Input: dimensioned drawing with shaded views. Units: mm. Origin: part minimum x, y, z. Coordinates: 2 decimals unless noted, no trailing zeros. Order: outer loops, then holes, each group sorted by start corner. A loop starts at its lowest first (then second) coordinate and runs counter-clockwise, first axis right, second up. Notation, with made-up numbers: (-4, 26) - (30, 26) arc R32 ccw to (30, 58) - close; hole circle Ø11 at (-27.5, -9). An arc over 180 degrees is marked (long way). Answer as CSV lines item,"result". Start each with the question number.
Item 1: Section C-C (x = 167). Output: boundary loops of the cut face in (y, z), and give its area (3 significant figures).
Item 2: Section B-B (z = 4). Output: boundary loops of the cut face in (x, y).
Item 3: Material intervals for line 1 along X through (y, z) = (57.5, 4); line 2 along Y through (x, z) = (75.5, 1), sorted ascending.
Item 4: First-contact query: pin 1 (6 mm diameter, centred on x = 26.5, y = 10.5, fed in from -Z); pin 2 (2.5 mm diameter, centred on y = 56, z = 2.5, fed in from -X); pin 3 (1.5 mm diameter, centred on y = 4.5, z = 3, fed in from +X); pin 4 (1.5 mm diameter, centred on x = 64.5, z = 3.5, fed in from +Y). Flat tips, straight axial feed; report the tip coordinate or a pass-through.
Item 5: Section A-A (y = 56). Output: boundary loops of the cut face in (x, z).
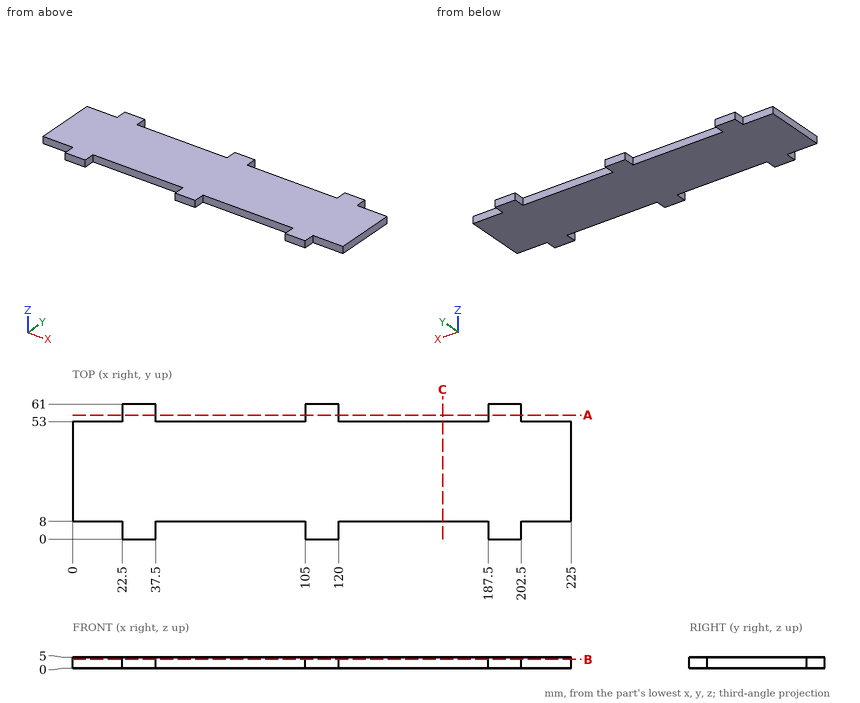
Determined:
1,outline,"(8, 0) - (53, 0) - (53, 5) - (8, 5) - close"
1,area,"225 mm^2"
2,outline,"(0, 8) - (22.5, 8) - (22.5, 0) - (37.5, 0) - (37.5, 8) - (105, 8) - (105, 0) - (120, 0) - (120, 8) - (187.5, 8) - (187.5, 0) - (202.5, 0) - (202.5, 8) - (225, 8) - (225, 53) - (202.5, 53) - (202.5, 61) - (187.5, 61) - (187.5, 53) - (120, 53) - (120, 61) - (105, 61) - (105, 53) - (37.5, 53) - (37.5, 61) - (22.5, 61) - (22.5, 53) - (0, 53) - close"
3,line 1,"x = 22.5 to 37.5, 105 to 120, 187.5 to 202.5"
3,line 2,"y = 8 to 53"
4,pin 1,"stops at z = 0"
4,pin 2,"stops at x = 22.5"
4,pin 3,"stops at x = 202.5"
4,pin 4,"stops at y = 53"
5,outline,"(22.5, 0) - (37.5, 0) - (37.5, 5) - (22.5, 5) - close; (105, 0) - (120, 0) - (120, 5) - (105, 5) - close; (187.5, 0) - (202.5, 0) - (202.5, 5) - (187.5, 5) - close"
